For this review, use the dimensioned drawing (mm, ordinates from the lowest corner) and the shaded views. A direction names the side the tool comes from. Coordinates: 2 decimals unless noted, no trailing zeros. Order: outer loops, then holes, each group sorted by start corner. A loop starts at its lowest first (then second) coordinate and runs counter-clockwise, first axis right, second up. Notation, with made-up numbers: (40.25, -16.75) -> (73.25, -16.75) arc R16 cw to (73.25, 7.25) -> close; hole circle Ø4 at (-31, -37.5). An arc over 180 degrees is marked (long way). Return JSON: item names as keys, results as strings. Group by question number.
Item 1: Take a section at D-D (x = 56). Write out the cut boundary in (y, z), then the cut area to 3 significant figures.
Item 2: Take a section at B-B (x = 29.9). Write out the cut boundary in (y, z).
Item 3: Insertion check: pin 1 (6 mm diameter, centred on x = 39, z = 60, fed in from -Y); pin 2 (13 mm diameter, centred on x = 29.9, z = 15.47, fed in from -Y); pin 3 (5 mm diameter, centred on y = 4, z = 63, fed in from -X); pin 4 (2 mm diameter, centred on y = 3.5, z = 64, fed in from +X). Each pin has a flat end and moves straight along its axis. Give the tip position at first contact, or say it passes through.
Item 4: For line 1 along Z through (x, y) = (5, 2); line 2 along X through (y, z) = (1.5, 7.5); line 3 along Y through (x, z) = (11, 75.5), list the stretches that pass through material, from the lowest coordinate up.
Item 5: Take a section at C-C (z = 16). Write out the cut boundary in (x, y).
Item 6: Draft analysis for pull direction Z (two halves, no side actions). For the marked faces 3, 4 and 5, state which applies: +Z half, -Z half, draft (parallel to the pull), parting line (faces both ways), or undercut.
Item 7: Take a section at A-A (y = 2.5). Write out the cut boundary in (x, z).
Item 8: Machinability: for the marked faces 1 and 2, which of the approach directions +Z, -Z, +X, -X, +Y, -Y give a long, thin tool a straight path to every point of the face, cutting with its end or side? Answer none if there is none.
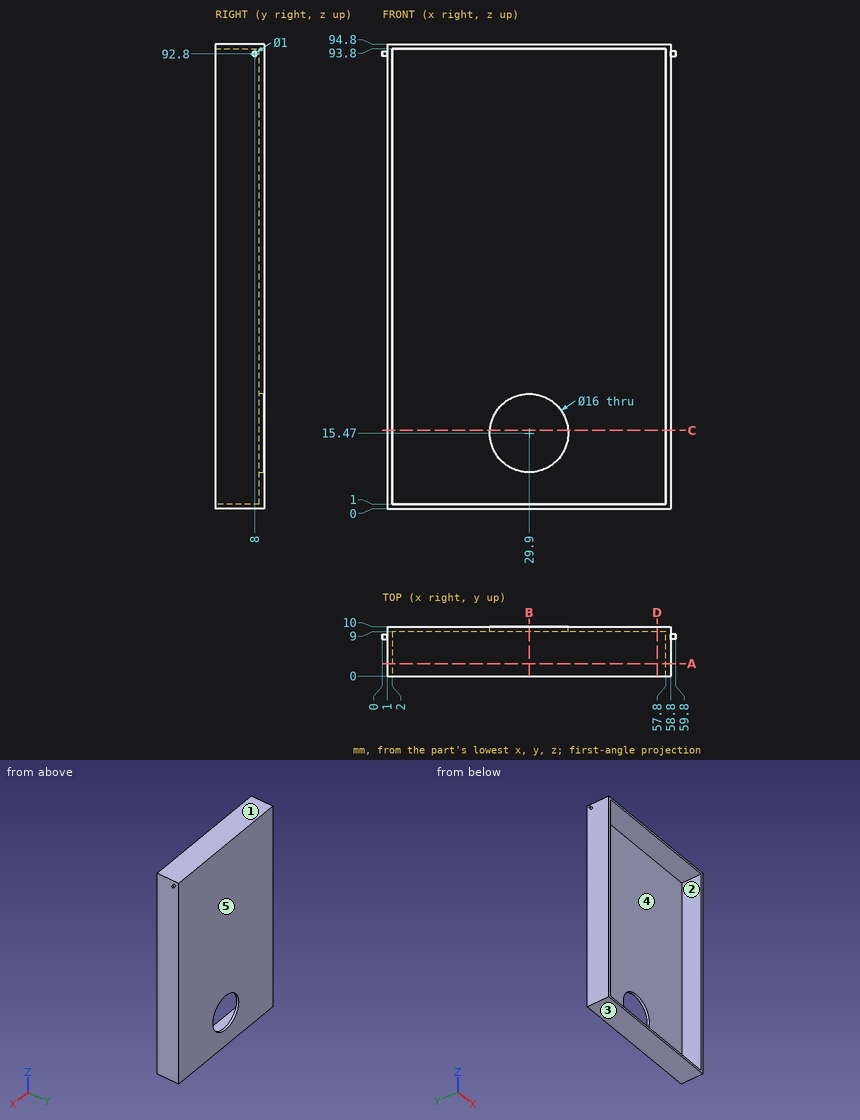
Findings below:
{
 "1": {"outline": "(0, 0) -> (10, 0) -> (10, 94.8) -> (0, 94.8) -> (0, 93.8) -> (9, 93.8) -> (9, 1) -> (0, 1) -> close", "area": "113 mm2"},
 "2": {"outline": "(0, 0) -> (10, 0) -> (10, 7.47) -> (9, 7.47) -> (9, 1) -> (0, 1) -> close; (0, 93.8) -> (9, 93.8) -> (9, 23.47) -> (10, 23.47) -> (10, 94.8) -> (0, 94.8) -> close"},
 "3": {"pin 1": "stops at y = 9", "pin 2": "passes through", "pin 3": "stops at x = 1", "pin 4": "stops at x = 58.8"},
 "4": {"line 1": "z = 0 to 1, 93.8 to 94.8", "line 2": "x = 1 to 2, 57.8 to 58.8", "line 3": "y = 9 to 10"},
 "5": {"outline": "(1, 0) -> (2, 0) -> (2, 9) -> (21.92, 9) -> (21.92, 10) -> (1, 10) -> close; (37.88, 9) -> (57.8, 9) -> (57.8, 0) -> (58.8, 0) -> (58.8, 10) -> (37.88, 10) -> close"},
 "6": {"face 3": "-Z half", "face 4": "undercut", "face 5": "draft"},
 "7": {"outline": "(1, 0) -> (58.8, 0) -> (58.8, 94.8) -> (1, 94.8) -> close; hole (2, 1) -> (57.8, 1) -> (57.8, 93.8) -> (2, 93.8) -> close"},
 "8": {"face 1": "+Z, +X, -X, +Y, -Y", "face 2": "-Y"}
}
